Here's how the part is built. I have some questions about the finished solid (model axes, mm). A direction names the side the tool comes from. Coordinates: 2 decimals unless noted, no trailing zeros. Write each loop counter-clockwise with the first axis right and the second up, starting at its lowest first coordinate (ties: lowest second). Pieces come first, ordered by that corner, then holes.
Item 1: I want a section at B-B (y = 59). Please give me the cut outline in (x, z).
Item 2: I want a section at D-D (y = -46.5). Please give me the cut outline in (x, z).
Item 3: If we mould it in two halves opening along Y, with no side actions, what happens to faces 1 (the face through (-82.5, -61, 10)), 2 (the face through (-69.119, 83.575, 10.028)), 3 (the face through (0, -98, 1))? For each: pulls with the +Y half, pulls with the -Y half, needs draft (parallel to the pull), parting line crosses it, or undercut.
Item 4: I want a section at C-C (x = -71.5). Please give me the cut outline in (y, z), and give its area (3 significant figures).
Item 5: For faces 4 (the face through (62.5, -1, 4)), 5 (the face through (5.3, 43.7, 1)), 6 (the face through (60.5, -1, 7)), which set-ups out of +Z, -Z, +X, -X, +Y, -Y let a thin tool reach every point of the face, with its end or its side?
Item 6: Please list where these lines run through material, in increasing order: line 1 (Y direction, x = 71.5, z = 9.7); line 2 (Y direction, x = -17.65, z = 0.45); line 3 (X direction, y = 76.5, z = 0.2).
Item 7: I'm going to push flat-ended pins straight in: P1, Ø3.5, axis at x = 71.5, y = -5.25, coming from the -Z side; P2, Ø4, axis at y = -19.5, z = 5.5, coming from the +X side; P3, Ø6, axis at x = -74.5, y = -51, coming from the -Z side; P4, Ø0.5, axis at y = 67.5, z = 1.5, coming from the -X side. Where does each tip first touch, or does it pass through?
Item 8: I want a section at A-A (z = 4.75). Please give me the cut outline in (x, y).
Autodesk Fusion 360 part; units mm, degrees
sketch "extrusion" plane through (0, 0, 0) normal (0, 1, 0) x (1, 0, 0)
  line L0 (-82.5, -8) -> (-62.5, -8)
  line L1 (-62.5, -8) -> (-62.5, 0)
  line L2 (-62.5, 0) -> (62.5, 0)
  line L3 (62.5, 0) -> (62.5, -8)
  line L4 (62.5, -8) -> (82.5, -8)
  line L5 (-60.5, -12) -> (-60.5, -2)
  line L6 (-60.5, -2) -> (60.5, -2)
  line L7 (60.5, -2) -> (60.5, -12)
  line L8 (-82.5, -12) -> (-60.5, -12)
  line L9 (60.5, -12) -> (82.5, -12)
  line L10 (-82.5, -8) -> (-82.5, -12)
  line L11 (82.5, -8) -> (82.5, -12)
  dimension "d1" = 125
  dimension "d2" = 8
  dimension "d3" = 20
  dimension "d4" = 8
  dimension "d5" = 20
extrude "Extrude1" add sketch "extrusion" along normal mid plane 196
sketch "top holes" plane through (0, 0, 12) normal (0, 0, 1) x (-1, 0, 0)
  circle A0 centre (71.5, -81.75) radius 3
  line L0 (82.5, -98) -> (60.5, -98)
  dimension "d11" = 6
  dimension "d12" = 16.25
extrude "Extrude2" cut sketch "top holes" against normal blind 4
mirror "Mirror1" about plane through (0, 0, 0) normal (1, 0, 0) of "Extrude2"
mirror "Mirror2" about plane through (0, 0, 0) normal (0, 1, 0) of "Extrude2", "Mirror1"
sketch "square undent" plane through (0, 0, 2) normal (0, 0, 1) x (-1, 0, 0)
  line L0 (22.5, -81.5) -> (-22.5, -81.5)
  line L1 (-22.5, -81.5) -> (-22.5, -36.5)
  line L2 (-22.5, -36.5) -> (22.5, -36.5)
  line L3 (22.5, -36.5) -> (22.5, -81.5)
  line L4 (60.5, -98) -> (-60.5, -98)
  dimension "d17" = 45
  dimension "d18" = 45
  dimension "d19" = 16.5
extrude "Extrude3" cut sketch "square undent" against normal blind 1
sketch "square holes" plane through (0, 0, 1) normal (0, 0, 1) x (-1, 0, 0)
  circle A0 centre (17.65, -76.5) radius 1.75
  line L0 (22.5, -81.5) -> (-22.5, -81.5)
  line L1 (22.5, -36.5) -> (22.5, -81.5)
  line L2 (-22.5, -36.5) -> (22.5, -81.5) construction
  circle A1 centre (0, -59) radius 16
  arc A2 (4.2359, -58.0006) -> (0, -43) centre (-16.1329, -55.654) ccw
  arc A3 (6.0614, -58.6697) -> (7.9315, -45.1043) centre (-7.0111, -49.9559) ccw
  arc A4 (4.2359, -58.0006) -> (6.0614, -58.6697) centre (5.2293, -58.115) ccw
  dimension "d22" = 3.5
  dimension "d23" = 5
  dimension "d24" = 4.85
  dimension "d25" = 32
  dimension "d26" = 1
  dimension "d35" = 5.2293
  dimension "d36" = 7.9315
  dimension "d37" = 15.7105
  dimension "d38" = 20.5035
  dimension "d39" = 0.885
extrude "Extrude4" cut sketch "square holes" against normal blind 1 contours A0
ref_plane "WorkPlane1" through (0, 59, 1.5) normal (0, -1, 0) x (-1, 0, 0)
mirror "Mirror3" about plane through (0, 59, 1.5) normal (0, -1, 0) of "Extrude4"
mirror "Mirror4" about plane through (0, 0, 0) normal (1, 0, 0) of "Extrude4", "Mirror3"
extrude "Extrude5" cut sketch "square holes" against normal blind 1 contours A1 A2 A3 A4 picked at (-1.7065, -54.7053)
pattern_circular "C-Pattern1" count 5 over 360 about axis through (0, 59, 1) along (0, 0, -1) of "Extrude5"
sketch "midhole" plane through (0, 0, 12) normal (0, 0, 1) x (-1, 0, 0)
  circle A0 centre (71.5, 5.25) radius 3
  circle A1 centre (71.5, -81.75) radius 3
  dimension "d40" = 81
extrude "Extrude6" cut sketch "midhole" against normal blind 4 contours A0
mirror "Mirror5" about plane through (0, 0, 0) normal (1, 0, 0) of "Extrude6"
sketch "Sketch6" plane through (0, 0, 12) normal (0, 0, 1) x (-1, 0, 0)
  line L0 (60.5, 22.5) -> (82.5, 22.5)
  line L1 (82.5, 22.5) -> (82.5, 17.5)
  line L2 (82.5, 17.5) -> (60.5, 17.5)
  line L3 (60.5, 17.5) -> (60.5, 22.5)
  line L4 (60.5, 98) -> (60.5, -98)
  line L5 (82.5, 98) -> (82.5, -98)
  line L6 (60.5, 98) -> (82.5, 98)
  dimension "d44" = 5
  dimension "d45" = 75.5
extrude "Extrude7" cut sketch "Sketch6" against normal blind 4 contours L0 L1 L2 L3 L4 L5
Answer:
1. outline: (-82.5, 8) - (-62.5, 8) - (-62.5, 0) - (-16, 0) - (-16, 1) - (-22.5, 1) - (-22.5, 2) - (-60.5, 2) - (-60.5, 12) - (-82.5, 12) - close; (16, 0) - (62.5, 0) - (62.5, 8) - (82.5, 8) - (82.5, 12) - (60.5, 12) - (60.5, 2) - (22.5, 2) - (22.5, 1) - (16, 1) - close
2. outline: (-82.5, 8) - (-62.5, 8) - (-62.5, 0) - (62.5, 0) - (62.5, 8) - (82.5, 8) - (82.5, 12) - (60.5, 12) - (60.5, 2) - (-60.5, 2) - (-60.5, 12) - (-82.5, 12) - close
3. face 1: needs draft
3. face 2: undercut
3. face 3: pulls with the -Y half
4. outline: (-98, 8) - (-84.75, 8) - (-84.75, 12) - (-98, 12) - close; (-78.75, 8) - (-22.5, 8) - (-22.5, 12) - (-78.75, 12) - close; (-17.5, 8) - (-8.25, 8) - (-8.25, 12) - (-17.5, 12) - close; (-2.25, 8) - (78.75, 8) - (78.75, 12) - (-2.25, 12) - close; (84.75, 8) - (98, 8) - (98, 12) - (84.75, 12) - close
4. area: 692 mm2
5. face 4: -Z, +X, +Y, -Y
5. face 5: +Z
5. face 6: +Z, +Y, -Y
6. line 1: y = -98 to -84.75, -78.75 to -8.25, -2.25 to 78.75, 84.75 to 98
6. line 2: y = -98 to 39.75, 43.25 to 74.75, 78.25 to 98
6. line 3: x = -62.5 to -19.4, -15.9 to 15.9, 19.4 to 62.5
7. P1: passes through
7. P2: stops at x = 62.5
7. P3: stops at z = 8
7. P4: stops at x = -62.5
8. outline: (-62.5, -98) - (-60.5, -98) - (-60.5, 98) - (-62.5, 98) - close; (60.5, -98) - (62.5, -98) - (62.5, 98) - (60.5, 98) - close
